```python
from build123d import *

# Parameters (mm, degrees)
SKETCH2_R          = 1
CUT_EXTRUDE1_DEPTH = 0.3
CHAMFER1_SIZE      = 0.3
SKETCH3_R          = 1
CUT_EXTRUDE2_DEPTH = 0.7


with BuildPart() as part:
    # Sketch1 → Revolve1 (revolve)
    with BuildSketch(Plane(origin=(0, 0, 0), x_dir=(1, 0, 0), z_dir=(0, 1, 0)), mode=Mode.PRIVATE) as revolve1_sk:
        Polygon((-7, 0), (-7, 2), (-6, 3), (0, 3), (0, 5), (9.8, 5), (15, 1.9977786), (15, 0), align=None)
    revolve(revolve1_sk.sketch.rotate(Axis((-2.845265589, 0, 0), (1, 0, 0)), 180), axis=Axis((-2.845265589, 0, 0), (1, 0, 0)))

    # Sketch2 → Cut-Extrude1 (cut)
    with BuildSketch(Plane(origin=(15, 0, 0), x_dir=(0, 0, -1), z_dir=(1, 0, 0))):
        Circle(SKETCH2_R)
    extrude(amount=-CUT_EXTRUDE1_DEPTH, mode=Mode.SUBTRACT)

    # Chamfer1
    chamfer1_edges = [part.edges().sort_by_distance(p)[0] for p in [
        (15, 0, 1),
    ]]
    chamfer(chamfer1_edges, length=CHAMFER1_SIZE - 0.0001)  # a hair under: the kernel refuses the full size

    # Sketch3 → Cut-Extrude2 (cut)
    with BuildSketch(Plane(origin=(14.7, 0, 0), x_dir=(0, 0, -1), z_dir=(1, 0, 0))):
        Circle(SKETCH3_R)
    extrude(amount=-CUT_EXTRUDE2_DEPTH, mode=Mode.SUBTRACT)

    # Cut-Extrude3 cone 1 section (through the dimple's axis) → Cut-Extrude3 (revolve, cut)
    with BuildSketch(Plane(origin=(14, 0, 0), x_dir=(0, 0, -1), z_dir=(0, 1, 0))):
        Polygon((0, 0), (1, 0), (0, 1), align=None)
    revolve(axis=Axis((14, 0, 0), (-1, 0, 0)), mode=Mode.SUBTRACT)


solid = part.part
```
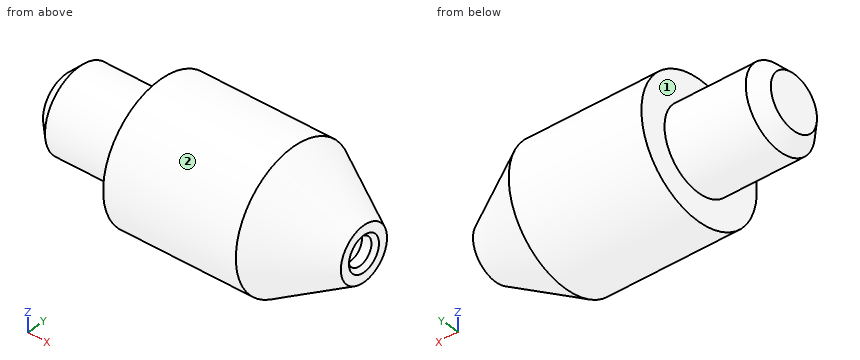
Model file for the job. Use its own axes, mm. Face numbers are marked on the shaded views. A direction names the side the tool comes from. Give positions to 0.01 mm unless a question says otherwise; leave off trailing zeros. Write each loop counter-clockwise with the first axis right and the second up, starting at its lowest first coordinate (ties: lowest second). Pieces come first, ordered by that corner, then holes. Notation, with made-up numbers: (0, 14) -> (41, 14) arc R25 cw to (41, 35) -> close; hole circle Ø11 at (-11, -11.5). An arc over 180 degrees is marked (long way). Use CSV: the item, a comma, the result in double quotes. Start each with the question number.
1) Tool access for the marked faces 1 and 2: list every direction of +Z, -Z, +X, -X, +Y, -Y with a clear straight run to the whole face (end or side of a thin tool).
2) Cut at C-C on x = 11. List the corners of the cut face in (y, z).
3) Pin check, flat tips, straight feed: P1, Ø6, axis at y = -3.5, z = -4, coming from the -X side; P2, Ø1, axis at x = -4, y = 0.5, coming from the -Z side; P3, Ø3, axis at y = -2, z = 3, coming from the +X side. Stop position of each tip, or through.
4) Cut at B-B on x = 13.25. List the corners of the cut face in (y, z), plus the area to 3 significant figures.
5) Drill centre lines: L1, parallel to Y at x = 14.25, z = 0; L2, parallel to Y at x = 14.2, z = 0; L3, parallel to Y at x = 9.75, z = 4. Where is each one in solid material? Low to high.
6) Cut at A-A on x = 3. List the corners of the cut face in (y, z), plus the area to 3 significant figures.
Final values:
1,face 1,"-X"
1,face 2,"+X, -X"
2,outline,"circle Ø8.61 at (0, 0)"
3,P1,"stops at x = -6.68"
3,P2,"stops at z = -3"
3,P3,"stops at x = 14.81"
4,outline,"circle Ø6.02 at (0, 0); hole circle Ø0.5 at (0, 0)"
4,area,"28.2 mm2"
5,L1,"y = -2.43 to -1, 1 to 2.43"
5,L2,"y = -2.46 to -1, 1 to 2.46"
5,L3,"y = -3 to 3"
6,outline,"circle Ø10 at (0, 0)"
6,area,"78.5 mm2"
